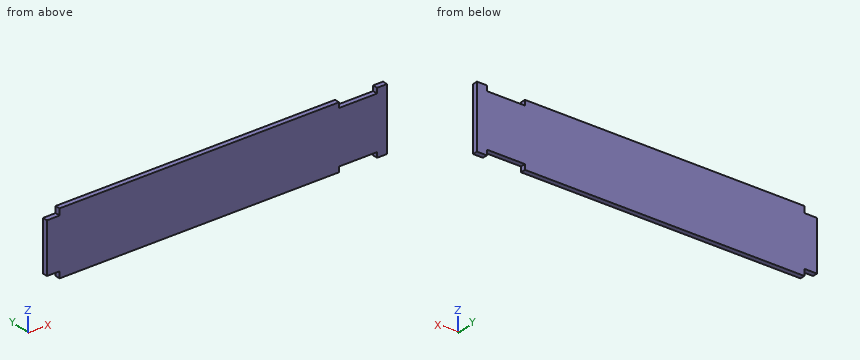
Autodesk Inventor part; units mm, degrees
ref_plane "YZ Plane" through (0, 0, 0) normal (1, 0, 0) x (0, 1, 0)
ref_plane "XZ Plane" through (0, 0, 0) normal (0, 1, 0) x (-1, 0, 0)
ref_plane "XY Plane" through (0, 0, 0) normal (0, 0, 1) x (1, 0, 0)
sketch "스케치1" plane through (0, 0, 0) normal (0, 1, 0) x (-1, 0, 0)
  line L0 (-199.7433, 25.7945) -> (-199.7433, -24.2055)
  line L1 (-149.7433, 25.7945) -> (-149.7433, -24.2055) construction
  line L2 (-161.6433, 25.7945) -> (-161.6433, 21.6945)
  line L3 (-161.6433, 21.6945) -> (-191.8433, 21.6945)
  line L4 (-191.8433, 21.6945) -> (-191.8433, 25.7945)
  line L5 (-153.7433, 25.7945) -> (-153.7433, -24.2055) construction
  line L6 (-161.6433, -24.2055) -> (-161.6433, -20.1055)
  line L7 (-161.6433, -20.1055) -> (-191.8433, -20.1055)
  line L8 (-191.8433, -20.1055) -> (-191.8433, -24.2055)
  line L9 (60.2567, 25.7945) -> (60.2567, 20.6945)
  line L10 (60.2567, 20.6945) -> (70.2567, 20.6945)
  line L11 (70.2567, 20.6945) -> (70.2567, -19.1055)
  line L12 (70.2567, -19.1055) -> (60.2567, -19.1055)
  line L13 (60.2567, -19.1055) -> (60.2567, -24.2055)
  line L14 (60.2567, -24.2055) -> (-161.6433, -24.2055)
  line L15 (-191.8433, -24.2055) -> (-199.7433, -24.2055)
  line L16 (60.2567, 25.7945) -> (-161.6433, 25.7945)
  line L17 (-191.8433, 25.7945) -> (-199.7433, 25.7945)
  point P0 (0, 0)
  point P1 (-199.7433, 0.7945)
  point P2 (-149.7433, 0.7945)
  point P3 (-161.6433, 23.7445)
  point P4 (-161.6433, -22.1555)
  point P5 (-195.7933, -24.2055)
  dimension "d2" = 260
  dimension "d4" = 50
  dimension "d5" = 4.1
  dimension "d6" = 30.2
  dimension "d7" = 4
  dimension "d8" = 7.9
  dimension "d9" = 4.1
  dimension "d10" = 30.2
  dimension "d11" = 7.9
  dimension "d12" = 5.1
  dimension "d13" = 5.1
  dimension "d14" = 10
  dimension "d17" = 50
extrude "돌출1" add sketch "스케치1" along normal blind 4
properties part number "우측 센서 막대기"
For this review, take the finished solid that the model builds, in its own axes (mm). Round coordinates to 2 decimals unless told otherwise and drop trailing zeros. Write each loop counter-clockwise with the first axis right and the second up, starting at its lowest first coordinate (ties: lowest second). Pieces come first, ordered by that corner, then holes. Notation, with made-up numbers: (-33.5, 88) - (8.5, 88) arc R11 ccw to (8.5, 98) - close; hole circle Ø8 at (-2, 61). An arc over 180 degrees is marked (long way). Use a Markdown table: item, result.
Q1. We need section B-B (x = 174.5). Give the boundary of the cut face in (y, z).
Derived:
| item | result |
|---|---|
| outline | (0, -20.11) - (4, -20.11) - (4, 21.69) - (0, 21.69) - close |
Q2. We need section A-A (y = 0.7). Give the boundary of the cut face in (x, z).
Derived:
| item | result |
|---|---|
| outline | (-70.26, -19.11) - (-60.26, -19.11) - (-60.26, -24.21) - (161.64, -24.21) - (161.64, -20.11) - (191.84, -20.11) - (191.84, -24.21) - (199.74, -24.21) - (199.74, 25.79) - (191.84, 25.79) - (191.84, 21.69) - (161.64, 21.69) - (161.64, 25.79) - (-60.26, 25.79) - (-60.26, 20.69) - (-70.26, 20.69) - close |
Q3. Clearance check with flat-ended pins moving along their axes: pin 1 (2 mm diameter, centred on x = -67.5, y = 2.5, fed in from -Z); pin 2 (1.2 mm diameter, centred on y = 3, z = 24, fed in from -X); pin 3 (2 mm diameter, centred on x = -63.5, y = 2, fed in from +Z). State where each tip first meets the part, or that it passes through.
Derived:
| item | result |
|---|---|
| pin 1 | stops at z = -19.11 |
| pin 2 | stops at x = -60.26 |
| pin 3 | stops at z = 20.69 |
Q4. Wall thickness on line 1 along X through (y, z) = (2.85, 22); line 2 along X through (y, z) = (1.1, 21); line 3 along Z through (x, y) = (189.5, 1.65): over which ranges is each line inside the solid? List them lowest first.
Derived:
| item | result |
|---|---|
| line 1 | x = -60.26 to 161.64, 191.84 to 199.74 |
| line 2 | x = -60.26 to 199.74 |
| line 3 | z = -20.11 to 21.69 |
